CAD build for the part. Positions are in the model's coordinates, mm. Face numbers are marked on the shaded views. A direction names the side the tool comes from. Give positions to 0.01 mm unless a question says otherwise; leave off trailing zeros. Write each loop counter-clockwise with the first axis right and the second up, starting at its lowest first coordinate (ties: lowest second). Pieces come first, ordered by that corner, then holes. Notation, with made-up numbers: M 4.25,21.5 L 25.25,21.5 A22 ccw 25.25,44.5 Z; hole C 8.5,49 d1. An arc over 180 degrees is marked long. One line per question, with ' | ' between items. Start each with the question number.
1. Which spindle directions (+Z, -Z, +X, -X, +Y, -Y) get a long thin tool onto all of the face, cutting with end or side? Do the marked faces 1 and 2. Say none if no direction does.
2. Cut at B-B, the plane z = 1. Count the separate pieces of the cut face and the enclosed holes in it, then the cut area to 3 significant figures.
3. Pull direction X, two halves, no side cores. Call the marked faces 3, 4, 5 and 6: released by +X, released by -X, zero draft, split by the parting line, or undercut.
4. Cut at A-A, the plane z = 7.5. Write the cut outline in (x, y).
5. Flat gauge pins, fed straight in: pin 1 (4 mm diameter, centred on x = -19.5, y = 5, fed in from +Z); pin 2 (3 mm diameter, centred on y = 13.5, z = 5, fed in from -X); pin 3 (4 mm diameter, centred on y = 3, z = -15, fed in from -X). Where does each tip first touch, or does it go through?
6. Wall check: L1, parallel to X at y = 13.5, z = -4.5; L2, parallel to X at y = 7.75, z = 4; L3, parallel to X at y = 17.5, z = 8. Give the ranges that are in metal, low to high.
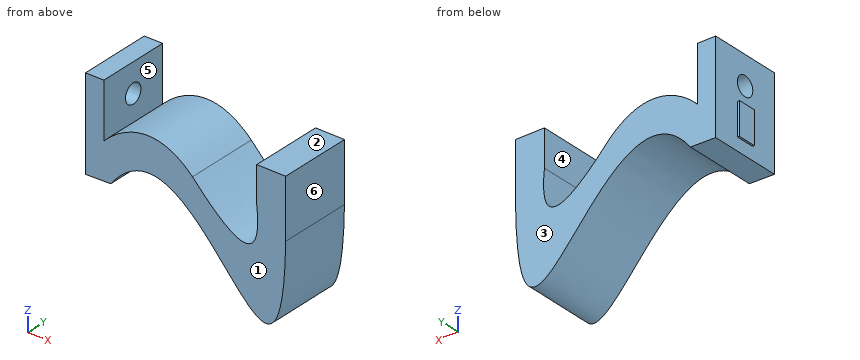
```python
from build123d import *

# Parameters (mm, degrees)
BOSS_EXTRUDE3_DEPTH = 20
SKETCH3_R           = 2.625
CUT_EXTRUDE1_DEPTH  = 6.0000001
SKETCH4_W           = 8.823264565
SKETCH4_H           = 5
BOSS_EXTRUDE4_DEPTH = 0.5


with BuildPart() as part:
    # Sketch1 → Boss-Extrude3 (new body)
    with BuildSketch(Plane(origin=(0, 0, 0), x_dir=(1, 0, 0), z_dir=(0, 1, 0))):
        with BuildLine():
            Line((-24.199448649, 0), (-24.199448649, -4.824773701))
            Line((-24.199448649, -4.824773701), (-24.199448649, -15.004197918))
            Line((-24.199448649, -15.004197918), (-29.199448649, -15.004197918))
            Line((-29.199448649, -15.004197918), (-29.199448649, -4.824773701))
            Line((-29.199448649, -4.824773701), (-29.199448649, 9.995802082))
            Line((-29.199448649, 9.995802082), (-22.322379413, 9.822250815))
            add(Edge.make_bspline(
                [(-22.322379413, 9.822250815), (0.232629534, -19.940907612), (24.467567917, 67.681570283), (25.436252045, 6.659493601)],
                knots=[0, 0, 0, 0, 1, 1, 1, 1], degree=3))
            Line((25.436252045, 6.659493601), (25.436252045, -9.362628557))
            Line((25.436252045, -9.362628557), (17.536308623, -9.362628557))
            Line((17.536308623, -9.362628557), (17.536308623, 0.546329))
            add(Edge.make_bspline(
                [(0, 0), (19.89900847, 21.841866163), (17.536308623, 0.546329)],
                knots=[0, 0, 0, 1, 1, 1], degree=2))
            add(Edge.make_bspline(
                [(-24.199448649, 0), (-24.197798481, -0.001931794), (-13.033999021, -12.890058665), (0, 0)],
                knots=[0, 0, 0, 0, 1, 1, 1, 1], degree=3))
        make_face()
    extrude(amount=BOSS_EXTRUDE3_DEPTH)

    # Sketch3 → Cut-Extrude1 (cut, through all)
    with BuildSketch(Plane(origin=(-24.199448649, 0, 0), x_dir=(0, 0, -1), z_dir=(1, 0, 0))):
        with Locations((-7.181936729, 10)):
            Circle(SKETCH3_R)
    extrude(amount=-CUT_EXTRUDE1_DEPTH, mode=Mode.SUBTRACT)

    # Sketch4 → Boss-Extrude4 (add)
    with BuildSketch(Plane.ZY.offset(29.199448649)):
        with Locations((-2.086858582, 10)):
            Rectangle(SKETCH4_W, SKETCH4_H)
    extrude(amount=BOSS_EXTRUDE4_DEPTH)


solid = part.part
```
Here are the results:
1) face 1: +Z, -Z, +X, -X, -Y | face 2: +Z, +X, +Y, -Y
2) separate pieces: 3 | enclosed holes: 0 | area: 703 mm^2
3) face 3: zero draft | face 4: undercut | face 5: undercut | face 6: released by +X
4) outline: M -29.2,0 L -24.2,0 L -24.2,7.39 L -29.2,7.39 Z; M -29.2,12.61 L -24.2,12.61 L -24.2,20 L -29.2,20 Z; M 17.54,0 L 25.44,0 L 25.44,20 L 17.54,20 Z
5) pin 1: z = 4.64 | pin 2: x = -29.2 | pin 3: x = 3.56
6) L1: -29.2 to -16.32, -7.2 to 4.33, 17.79 to 25.44 | L2: -29.2 to -24.2, -18.9 to -5.33, 17.54 to 25.44 | L3: -29.2 to -24.2, 17.54 to 25.44
